from build123d import *

# Parameters (mm, degrees)
F0_R     = 38.6580677432
F1_DEPTH = 60.7483312488
F2_DEPTH = 25.4
F3_DEPTH = 25.4


with BuildPart() as f1:
    # F0 (on Top) → F1 (new body)
    with BuildSketch(Plane.XY):
        with Locations((0.5874064986, -0.0370815396)):
            Circle(F0_R)
    extrude(amount=F1_DEPTH)

    # F2 (add): a face of the model
    f2_faces = [f1.faces().sort_by_distance(p)[0] for p in [
        (0.5874064986, -0.0370815396, 60.7483312488),
    ]]
    extrude(f2_faces, amount=F2_DEPTH)

    # F3 (add): a face of the model
    f3_faces = [f1.faces().sort_by_distance(p)[0] for p in [
        (0.5874064986, -0.0370815396, 86.1483312488),
    ]]
    extrude(f3_faces, amount=F3_DEPTH)


solid = f1.part
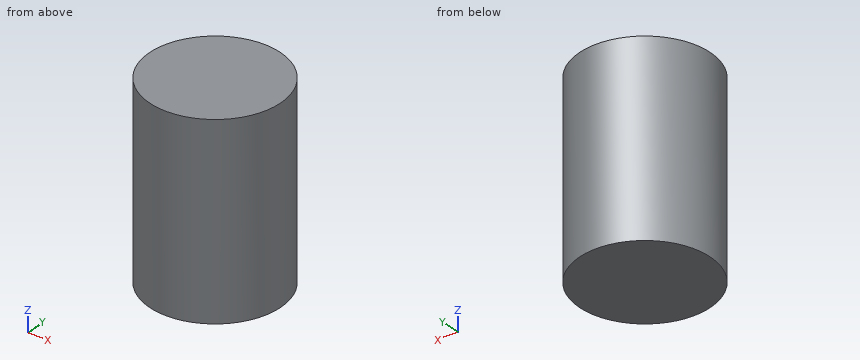
Could you check a few things on this model? Use its own coordinates, in mm. Round coordinates to 2 decimals unless told otherwise and drop trailing zeros. Order: outer loops, then holes, each group sorted by start corner. A loop starts at its lowest first (then second) coordinate and runs counter-clockwise, first axis right, second up. Notation, with made-up numbers: M 17,-32.75 L 46,-32.75 A21 ccw 46,5.25 Z; hole C 4,18.25 d5. An arc over 180 degrees is marked long. One line per item, written item: value.
(1) Imagine slicing it at C-C (z = 66). Write out the boundary of the cut face in (x, y).
Ans:
outline: C 0.59,-0.04 d77.32
(2) Imagine slicing it at B-B (x = -24.5). Write out the boundary of the cut face in (y, z).
Ans:
outline: M -29.45,0 L 29.37,0 L 29.37,111.55 L -29.45,111.55 Z
(3) I need wall thicknesses on line 1 along Y through (x, z) = (1.5, 8); line 2 along X through (y, z) = (-13.5, 36.5); line 3 along X through (y, z) = (-23.5, 87.5). Which ranges of each line are inside material? Lowest first, please. Write a range as from..to.
Ans:
line 1: y = -38.68..38.61
line 2: x = -35.65..36.83
line 3: x = -30.14..31.31
(4) I'm going to push flat-ended pins straight in: P1, Ø4, axis at y = 2, z = 47, coming from the +X side; P2, Ø10, axis at x = 12, z = 37, coming from the +Y side; P3, Ø1.5, axis at y = -25, z = 44.5, coming from the +X side; P4, Ø6, axis at y = -7, z = 86, coming from the -X side. Where does each tip first touch, or does it pass through?
Ans:
P1: stops at x = 39.25
P2: stops at y = 38.09
P3: stops at x = 30.72
P4: stops at x = -37.87
(5) Imagine slicing it at A-A (y = -32). Write out the boundary of the cut face in (x, z).
Ans:
outline: M -21.16,0 L 22.33,0 L 22.33,111.55 L -21.16,111.55 Z
